Can you work these out from the model? Positions are in its coordinate system, mm. Face numbers are marked on the shaded views. A direction names the side the tool comes from. Give positions to 0.01 mm unless a question says otherwise; leave off trailing zeros. Order: outer loops, then holes, each group sorted by start corner. A loop starts at its lowest first (then second) coordinate and runs counter-clockwise, first axis right, second up. Notation, with made-up numbers: M -32,46 L 21,46 A31 cw 21,75 Z; hole C 78,-15.5 d7. An arc over 180 degrees is marked long. Answer as a JSON object with one key per item and string values.
```python
from build123d import *

# Parameters (mm, degrees)
F0_W      = 57.15
F0_H      = 31.75
F1_DEPTH  = 38.1
F3_DEPTH  = 12.7
F5_DEPTH  = 25.4
F6_DEPTH  = 12.7
F7_DEPTH  = 25.4
F9_DEPTH  = 25.4
F11_DEPTH = 50.8


with BuildPart() as f1:
    # F0 (on Front) → F1 (new body)
    with BuildSketch(Plane.XZ):
        with Locations((-1.4262031764, 0.0904835914)):
            Rectangle(F0_W, F0_H)
    extrude(amount=F1_DEPTH)

    # F2 (on face) → F3 (cut)
    with BuildSketch(Plane.XZ.offset(38.1)):
        Polygon((27.1487968236, 15.9654835914), (-10.9512031764, 15.9654835914), (1.7487968236, -15.7845164086), (27.1487968236, -15.7845164086), align=None)
    extrude(amount=-F3_DEPTH, mode=Mode.SUBTRACT)

    # F4 (on face) → F5 (join)
    with BuildSketch(Plane(origin=(0, 0, 0), x_dir=(-1, 0, 0), z_dir=(0, 1, 0))):
        Polygon((4.6012031764, -15.7845164086), (10.9512031764, 15.9654835914), (-27.1487968236, 15.9654835914), (-27.1487968236, -15.7845164086), align=None)
    extrude(amount=F5_DEPTH)

    # F6 (cut): a face of the model
    f6_faces = [f1.faces().sort_by_distance(p)[0] for p in [
        (9.638190763, 25.4, 0.5715441975),
    ]]
    extrude(f6_faces, amount=-F6_DEPTH, mode=Mode.SUBTRACT)

    # F7 (add): a face of the model
    f7_faces = [f1.faces().sort_by_distance(p)[0] for p in [
        (-18.8131079383, 0, -0.6654687896),
    ]]
    extrude(f7_faces, amount=F7_DEPTH)

    # F8 (on face) → F9 (cut)
    with BuildSketch(Plane.XZ.offset(25.4)):
        Polygon((27.1487968236, 15.9654835914), (14.4487968236, 15.9654835914), (27.1487968236, -15.7845164086), align=None)
    extrude(amount=-F9_DEPTH, mode=Mode.SUBTRACT)

    # F10 (on face) → F11 (cut)
    with BuildSketch(Plane(origin=(0, 12.7, 0), x_dir=(-1, 0, 0), z_dir=(0, 1, 0))):
        Polygon((-27.1487968236, -15.7845164086), (-1.7487968236, 15.9654835914), (-27.1487968236, 15.9654835914), align=None)
    extrude(amount=-F11_DEPTH, mode=Mode.SUBTRACT)


solid = f1.part
```
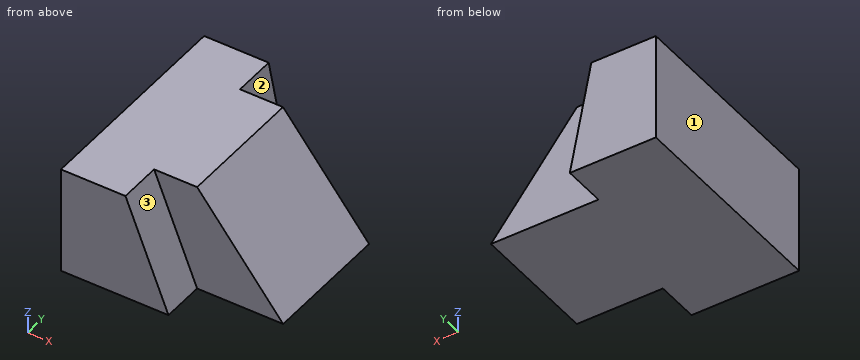
1) I want a section at C-C on y = -30. Write out the boundary of the cut face in (x, z).
Results found:
{"outline": "M -30,-15.78 L 1.75,-15.78 L -10.95,15.97 L -30,15.97 Z"}
2) I want a section at A-A on z = 1. Write out the boundary of the cut face in (x, y) (3 decimals), and give its area (3 significant figures).
Results found:
{"outline": "M -30.001,-38.1 L -4.965,-38.1 L -4.965,-25.4 L 13.721,-25.4 L 13.721,12.7 L -7.958,12.7 L -7.958,25.4 L -30.001,25.4 Z", "area": "2,260 mm²"}
3) I want a section at B-B on x = -6. Write out the boundary of the cut face in (y, z), and give its area (3 significant figures).
Results found:
{"outline": "M -38.1,-15.78 L 25.4,-15.78 L 25.4,-8.79 L 12.7,-8.79 L 12.7,15.97 L -25.4,15.97 L -25.4,3.59 L -38.1,3.59 Z", "area": "1,540 mm²"}
4) For the marked faces 1, 2 and 3, which set-ups out of +Z, -Z, +X, -X, +Y, -Y let a thin tool reach every point of the face, with its end or its side?
Results found:
{"face 1": "+Z, -Z, -X, +Y, -Y", "face 2": "+Z, +X, +Y", "face 3": "+Z, +X, -Y"}
5) I want a section at D-D on y = -21.5. Write out the boundary of the cut face in (x, z).
Results found:
{"outline": "M -30,-15.78 L 27.15,-15.78 L 1.75,15.97 L -30,15.97 Z"}
6) I need wall thicknesses on L1, parallel to Y at x = -3, z = 3; L2, parallel to Y at x = -2.5, z = -12.5; L3, parallel to X at y = -14.5, z = 7. Which ranges of each line are inside material? Lowest first, please.
Results found:
{"L1": "y = -25.4 to 12.7", "L2": "y = -38.1 to 12.7", "L3": "x = -30 to 8.92"}
7) I'm going to push flat-ended pins straight in: pin 1 Ø3 at (x, y) = (3.5, -13.5) entering from +Z; pin 2 Ø1 at (y, z) = (-1.5, -12.5) entering from +X; pin 3 Ø9.5 at (x, z) = (16.5, 3.5) entering from +Y. Where does each tip first touch, or does it pass through?
Results found:
{"pin 1": "stops at z = 15.65", "pin 2": "stops at x = 24.92", "pin 3": "stops at y = 12.7"}
